Verification items for the finished model (mm, model axes). A direction names the side the tool comes from. Coordinates: 2 decimals unless noted, no trailing zeros. Order: outer loops, then holes, each group sorted by start corner. A loop starts at its lowest first (then second) coordinate and runs counter-clockwise, first axis right, second up. Notation, with made-up numbers: (1.25, 6) - (60.25, 6) arc R16 ccw to (60.25, 30) - close; hole circle Ø10 at (28, -23.5). An arc over 180 degrees is marked (long way). One line per question, with ' | ' between items. Start each with the question number.
from build123d import *

# Parameters (mm, degrees)
F1_DEPTH = 38.1
F3_DEPTH = 25.4


with BuildPart() as f1:
    # F0 (on Top) → F1 (new body)
    with BuildSketch(Plane.XY):
        with BuildLine():
            ThreePointArc((-101.6, 175.976362), (203.2, 0), (-101.6, -175.976362))
            Line((-101.6, -175.976362), (-146.05, -252.96602))
            ThreePointArc((-146.05, -252.96602), (292.1, 0), (-146.05, 252.96602))
            Line((-146.05, 252.96602), (-101.6, 175.976362))
        make_face()
    extrude(amount=F1_DEPTH)

    # F2 (on face) → F3 (cut)
    with BuildSketch(Plane.XY.offset(38.1)):
        with BuildLine():
            ThreePointArc((-67.447957, 218.423289), (228.6, 0), (-67.447957, -218.423289))
            Line((-67.447957, -218.423289), (-72.327528, -226.874953))
            ThreePointArc((-72.327528, -226.874953), (238.125, 0), (-72.327528, 226.874953))
            Line((-72.327528, 226.874953), (-67.447957, 218.423289))
        make_face()
        with BuildLine():
            ThreePointArc((-86.914513, 252.140353), (266.7, 0), (-86.914513, -252.140353))
            Line((-86.914513, -252.140353), (-91.762687, -260.537636))
            ThreePointArc((-91.762687, -260.537636), (276.225, 0), (-91.762687, 260.537636))
            Line((-91.762687, 260.537636), (-86.914513, 252.140353))
        make_face()
    extrude(amount=-F3_DEPTH, mode=Mode.SUBTRACT)


solid = f1.part
Item 1: Section check A-A (z = 28.5). Record the cut outline in (x, y) (3 decimals), then the cut area to 3 significant figures.
Item 2: Section check C-C (y = 0). Record the cut outline in (x, z) (3 decimals), then the cut area to 3 significant figures.
Item 3: Section check D-D (x = 131). Record the cut outline in (y, z), then the cut area to 3 significant figures.
Item 4: Set-up check for faces 1 (the flat face through (216, 4, 0)), 2 (the flat face through (-124.136, 215.01, 18.783)), 3 (the cylindrical face through (276.126, -7.383, 25.578)): record each of +Z, -Z, +X, -X, +Y, -Y from which the full face is reachable in a straight line by a thin tool's end or side.
Item 5: Mould release check, pull along X, two halves, no side actions. Record for faces 4 (the flat face through (-123.514, -213.932, 18.783)), 5 (the flat face through (202, -42, 38.1)), 6 (the cylindrical face through (203.113, 5.957, 18.783)), 7 (the cylindrical face through (238.043, -6.265, 25.578)): +X half, -X half, draft (parallel to the pull), parting line (faces both ways), or undercut.
Item 6: Section check B-B (x = 0). Record the cut outline in (y, z) (3 decimals), then the cut area to 3 significant figures.
Item 7: Thickness scan on probe 1 along Y at (x, z) = (0, 13) (3 decimals); probe 2 along Y at (x, z) = (-40.5, 15); probe 3 along X at (y, z) = (-103.5, 36). Record the ranges inside material, lowest first. Write a range as from..to.
Item 8: Gauge pin test, flat ends, axial feed: pin 1 (2 mm diameter, centred on y = 177.5, z = 31.5, fed in from +X); pin 2 (3 mm diameter, centred on y = -208, z = 21, fed in from +X); pin 3 (8 mm diameter, centred on x = -67.5, z = 17.5, fed in from +Y). Record the tip position at first contact, or that the pin passes through.
Completed:
1) outline: (-146.05, -252.966) arc R292.1 ccw (long way) to (-146.05, 252.966) - (-101.6, 175.976) arc R203.2 cw (long way) to (-101.6, -175.976) - close; hole (-91.763, -260.538) arc R276.225 ccw (long way) to (-91.763, 260.538) - (-86.915, 252.14) arc R266.7 cw (long way) to (-86.915, -252.14) - close; hole (-72.328, -226.875) arc R238.125 ccw (long way) to (-72.328, 226.875) - (-67.448, 218.423) arc R228.6 cw (long way) to (-67.448, -218.423) - close | area: 74,000 mm^2
2) outline: (203.2, 0) - (292.1, 0) - (292.1, 38.1) - (276.225, 38.1) - (276.225, 12.7) - (266.7, 12.7) - (266.7, 38.1) - (238.125, 38.1) - (238.125, 12.7) - (228.6, 12.7) - (228.6, 38.1) - (203.2, 38.1) - close | area: 2,900 mm^2
3) outline: (-261.08, 0) - (-155.34, 0) - (-155.34, 38.1) - (-187.34, 38.1) - (-187.34, 12.7) - (-198.85, 12.7) - (-198.85, 38.1) - (-232.31, 38.1) - (-232.31, 12.7) - (-243.19, 12.7) - (-243.19, 38.1) - (-261.08, 38.1) - close; (155.34, 0) - (261.08, 0) - (261.08, 38.1) - (243.19, 38.1) - (243.19, 12.7) - (232.31, 12.7) - (232.31, 38.1) - (198.85, 38.1) - (198.85, 12.7) - (187.34, 12.7) - (187.34, 38.1) - (155.34, 38.1) - close | area: 6,920 mm^2
4) face 1: -Z, +X, -X, +Y, -Y | face 2: +Z, -Z, -X | face 3: +Z
5) face 4: -X half | face 5: draft | face 6: undercut | face 7: undercut
6) outline: (-292.1, 0) - (-203.2, 0) - (-203.2, 38.1) - (-228.6, 38.1) - (-228.6, 12.7) - (-238.125, 12.7) - (-238.125, 38.1) - (-266.7, 38.1) - (-266.7, 12.7) - (-276.225, 12.7) - (-276.225, 38.1) - (-292.1, 38.1) - close; (203.2, 0) - (292.1, 0) - (292.1, 38.1) - (276.225, 38.1) - (276.225, 12.7) - (266.7, 12.7) - (266.7, 38.1) - (238.125, 38.1) - (238.125, 12.7) - (228.6, 12.7) - (228.6, 38.1) - (203.2, 38.1) - close | area: 5,810 mm^2
7) probe 1: y = -292.1..-276.225, -266.7..-238.125, -228.6..-203.2, 203.2..228.6, 238.125..266.7, 276.225..292.1 | probe 2: y = -289.28..-273.24, -263.61..-234.66, -224.98..-199.12, 199.12..224.98, 234.66..263.61, 273.24..289.28 | probe 3: x = 174.87..203.83, 214.46..245.8, 256.1..273.15
8) pin 1: stops at x = 232.74 | pin 2: stops at x = 206.59 | pin 3: stops at y = 285.11
